CAD build for the part. Positions are in the model's coordinates, mm. A direction names the side the tool comes from. Give positions to 0.01 mm unless a question says otherwise; leave off trailing zeros. Order: outer loops, then holes, each group sorted by start corner. A loop starts at its lowest first (then second) coordinate and runs counter-clockwise, first axis right, second up. Notation, with made-up numbers: (82, 28) -> (140, 28) arc R20 ccw to (140, 47) -> close; hole circle Ø10 at (-0.75, 41). An arc over 180 degrees is marked (long way). Use one line per item in the form item = value. Start each with the question number.
1) Cut at A-A, the plane x = -0.9. Give the cut face in (y, z) (1 decimal).
2) Cut at C-C, the plane y = 12.5. Give the cut face in (x, z) (3 decimals).
3) Tool access for faces 5 (the face through (-3, 4, -9.025)), 6 (the face through (-1, 7.62, -13)), 7 (the face through (-3, 4, -110.625)): list every direction of +Z, -Z, +X, -X, +Y, -Y with a clear straight run to the whole face (end or side of a thin tool).
4) Drop flat-ended pins along their axis: P1, Ø2, axis at x = -3, y = 5, coming from the +Z side (3 decimals); P2, Ø8.5, axis at y = 5, z = -3.5, coming from the +X side; P3, Ø0.6, axis at x = 1, y = 2.5, coming from the -Z side (3 decimals). Give the stop position or say it passes through.
5) Cut at D-D, the plane z = -93. Give the cut face in (x, y) (3 decimals), and give its area (3 significant figures).
6) Cut at B-B, the plane y = 3.81. Give the cut face in (x, z) (3 decimals).
7) Mould opens along Z. For faces 1 (the face through (-0.912, 15.875, -59.291)), 2 (the face through (1, 4, -110.625)), 3 (the face through (1.905, 7, -59)), 4 (the face through (-0.94, 3.88, -113.55)) say: pulls with the +Z half, pulls with the -Z half, needs draft (parallel to the pull), parting line crosses it, or undercut.
8) Probe line 1 (Z direction, x = -2.55, y = 6) (3 decimals); line 2 (Y direction, x = -3.4, z = -57); line 3 (Z direction, x = -0.75, y = 9) (3 decimals). List the from-to ranges inside material, lowest first.
Autodesk Inventor part; units mm, degrees
ref_plane "YZ Plane" through (0, 0, 0) normal (1, 0, 0) x (0, 1, 0)
ref_plane "XZ Plane" through (0, 0, 0) normal (0, 1, 0) x (-1, 0, 0)
ref_plane "XY Plane" through (0, 0, 0) normal (0, 0, 1) x (1, 0, 0)
sketch "Sketch1" plane through (0, 0, 0) normal (0, 1, 0) x (-1, 0, 0)
  line L0 (0, 0) -> (1.905, 0)
  line L1 (1.905, -119.6501) -> (0, -119.6501)
  line L2 (0, 0) -> (0, -9.025)
  line L3 (0, 0) -> (9.025, 0) construction
  line L4 (0, -9.025) -> (1.905, -9.025)
  line L5 (0, -119.6501) -> (0, -110.625)
  line L6 (0, -110.625) -> (1.905, -110.625)
  line L7 (1.905, -9.025) -> (3.81, -9.025)
  line L8 (3.81, -9.025) -> (3.81, -110.625)
  line L9 (3.81, -110.625) -> (1.905, -110.625)
  line L10 (0, -9.025) -> (-1.905, -9.025)
  line L11 (-1.905, -9.025) -> (-1.905, -110.625)
  line L12 (-1.905, -110.625) -> (0, -110.625)
  line L13 (1.905, 0) -> (1.905, -9.025)
  line L14 (1.905, -110.625) -> (1.905, -119.6501)
  line L15 (0, -119.6501) -> (0, -110.625)
  line L16 (0, -9.025) -> (0, 0)
  dimension "d19" = 101.6
  dimension "d20" = 1.905
  dimension "d21" = 1.905
  dimension "d22" = 1.905
  dimension "d23" = 1.905
  dimension "d24" = 1.905
  dimension "d25" = 1.905
extrude "Extrusion1" add sketch "Sketch1" along normal blind 7.62 contours L0 L13 L4 L2 | L6 L14 L1 L5
extrude "Extrusion2" add sketch "Sketch1" along normal blind 19.05 contours L4 L7 L8 L9 L6 L12 L11 L10
sketch "Sketch2" plane through (0, 0, 0) normal (1, 0, 0) x (0, 0, -1)
  line L0 (9.025, 7.62) -> (0, 7.62)
  line L1 (4.5125, 7.62) -> (4.5125, 3.81)
  line L2 (0, 0) -> (0, 7.62)
  line L3 (9.025, 19.05) -> (110.625, 19.05)
  line L4 (59.825, 19.05) -> (59.825, 0)
  line L5 (9.025, 0) -> (110.625, 0)
  circle A0 centre (4.5125, 3.81) radius 1.5875
  circle A1 centre (115.1376, 3.81) radius 1.5875
  dimension "d12" = 3.175
extrude "Extrusion3" cut sketch "Sketch2" against normal blind 12.7
sketch "Sketch3" plane through (1.905, 0, -9.025) normal (1, 0, 0) x (0, 0, -1)
  line L0 (0, 19.05) -> (101.6, 19.05)
  line L1 (50.8, 19.05) -> (50.8, 15.875)
  arc A0 (0, 19.05) -> (101.6, 19.05) centre (50.8, 423.8625) ccw
  point P0 (-9.025, 0)
  dimension "d15" = 3.175
extrude "Extrusion4" cut sketch "Sketch3" against normal blind 12.7
fillet "Fillet1" radius 4.445 2 edges at (-0.9525, 19.05, -9.025) (-0.9525, 19.05, -110.625)
sketch "Sketch4" plane through (1.905, 0, -9.025) normal (1, 0, 0) x (0, 0, -1)
  line L0 (0, 0) -> (0, 7.62)
  line L1 (0, 7.62) -> (12.7, 7.62)
  line L2 (12.7, 7.62) -> (12.7, 20.32)
  line L3 (12.7, 20.32) -> (0, 20.32)
  line L4 (0, 20.32) -> (0, 7.62)
  line L5 (110.625, 7.62) -> (101.6, 7.62)
  line L6 (101.6, 7.62) -> (88.9, 7.62)
  line L7 (88.9, 7.62) -> (88.9, 20.32)
  line L8 (88.9, 20.32) -> (101.6, 20.32)
  line L9 (101.6, 20.32) -> (101.6, 7.62)
  point P0 (-9.025, 0)
  dimension "d26" = 12.7
  dimension "d27" = 12.7
  dimension "d28" = 12.7
  dimension "d29" = 12.7
extrude "Extrusion5" cut sketch "Sketch4" against normal blind 25.4
properties part number "FretBar"
Result:
q1.outline = (0, -119.7) -> (7.6, -119.7) -> (7.6, -97.9) -> (17.7, -97.9) arc R408 cw to (17.7, -21.7) -> (7.6, -21.7) -> (7.6, 0) -> (0, 0) -> close; hole circle Ø3.2 at (3.8, -115.1); hole circle Ø3.2 at (3.8, -4.5)
q2.outline = (-3.81, -97.925) -> (1.905, -97.925) -> (1.905, -21.725) -> (-3.81, -21.725) -> close
q3.face_5 = +Z, -X, +Y, -Y
q3.face_6 = +Z, +X, -X, +Y
q3.face_7 = -Z, -X, +Y, -Y
q4.P1 = -9.025
q4.P2 = 0
q4.P3 = -110.625
q5.outline = (-3.81, 0) -> (1.905, 0) -> (1.905, 17.226) -> (-3.81, 17.226) -> close
q5.area = 98.4 mm²
q6.outline = (-3.81, -110.625) -> (-1.905, -110.625) -> (-1.905, -113.55) -> (0, -113.55) -> (0, -110.625) -> (1.905, -110.625) -> (1.905, -9.025) -> (0, -9.025) -> (0, -6.1) -> (-1.905, -6.1) -> (-1.905, -9.025) -> (-3.81, -9.025) -> close; (-1.905, -119.65) -> (0, -119.65) -> (0, -116.725) -> (-1.905, -116.725) -> close; (-1.905, -2.925) -> (0, -2.925) -> (0, 0) -> (-1.905, 0) -> close
q7.face_1 = undercut
q7.face_2 = pulls with the -Z half
q7.face_3 = needs draft
q7.face_4 = undercut
q8.line_1 = -110.625 to -9.025
q8.line_2 = 0 to 15.88
q8.line_3 = -97.925 to -21.725
